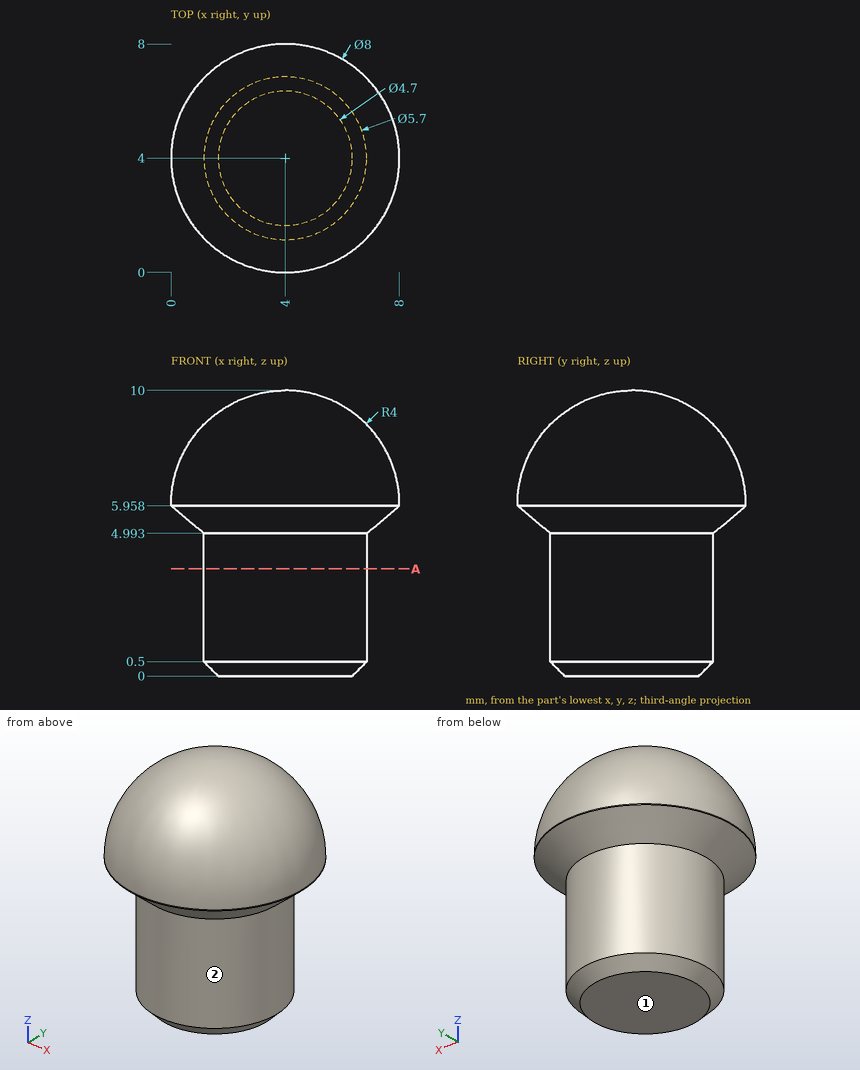
Check sheet for the drawn part. Datum: minimum x, y, z corner. Units: mm. A direction names the side the tool comes from. Round coordinates to 2 decimals unless told otherwise and drop trailing zeros. Order: outer loops, then holes, each group sorted by start corner. A loop starts at its lowest first (then second) coordinate and runs counter-clockwise, first axis right, second up.
(1) Go/stop test with flat-tipped pins: P1, Ø3, axis at x = 7, z = 9, coming from the -Y side; P2, Ø1, axis at x = 6, y = 6.5, coming from the -Z side; P3, Ø2, axis at x = 7, y = 3.5, coming from the +Z side. Record where each tip stops, or that it passes through.
(2) Cross-section at A-A, the plane z = 3.75. Enter the section's corners in (x, y).
(3) Access from +Z, -Z, +X, -X, +Y, -Y to the whole of each face (thin tool, end or side, straight path). Record for the marked faces 1 and 2.
(4) Scan lines: probe 1 along Y at (x, z) = (4.75, 5.75); probe 2 along Y at (x, z) = (4, 2.5). Record each from-to range of solid material in increasing order.
Check sheet entries:
1. P1: stops at y = 1.09
1. P2: stops at z = 0.35
1. P3: stops at z = 9.44
2. outline: circle Ø5.7 at (4, 4)
3. face 1: -Z, +X, -X, +Y, -Y
3. face 2: -Z
4. probe 1: y = 0.32 to 7.68
4. probe 2: y = 1.15 to 6.85
